Geometry: final body of the model. Coordinates: model frame, mm. Face numbers are marked on the shaded views. A direction names the side the tool comes from. Round coordinates to 2 decimals unless told otherwise and drop trailing zeros. Loops run counter-clockwise (first coordinate to the right, second up) from the corner with the lowest first, then second, coordinate; pieces in that order, holes last. Notation, with made-up numbers: M 82,43 L 119,43 A17 cw 119,59 Z; hole C 44,37 d5. An arc over 180 degrees is marked long. Write each question's results on one line, items separated by ' | '.
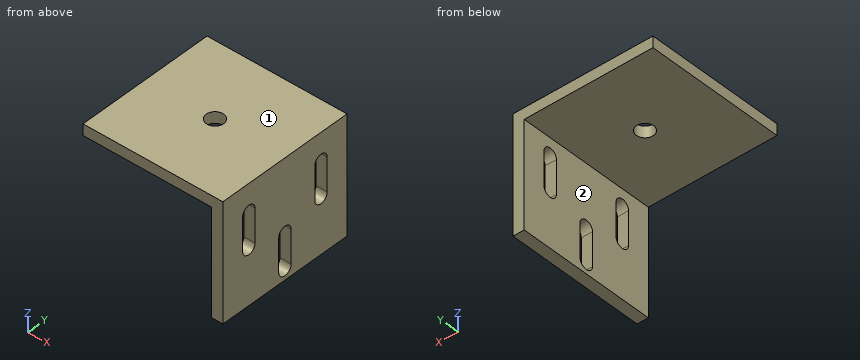
```python
from build123d import *

# Parameters (mm, degrees)
F1_DEPTH = 25
F3_D     = 6.2
F5_DEPTH = 4.001


with BuildPart() as f1:
    # F0 (on Front) → F1 (new body, symmetric)
    with BuildSketch(Plane.XZ):
        Polygon((0, -42), (0, 0), (-50, 0), (-50, -4), (-4, -4), (-4, -42), align=None)
    extrude(amount=F1_DEPTH, both=True)

    # F3 (through all)
    with Locations(Plane.XY):
        with Locations((-25, 0)):
            Hole(F3_D / 2)

    # F4 (on face) → F5 (cut, through all)
    with BuildSketch(Plane(origin=(-4, 0, 0), x_dir=(0, -1, 0), z_dir=(-1, 0, 0))):
        with BuildLine():
            ThreePointArc((-17.034974, -22), (-14.534974, -24.5), (-12.034974, -22))
            Line((-12.034974, -22), (-12.034974, -10))
            ThreePointArc((-12.034974, -10), (-14.534974, -7.5), (-17.034974, -10))
            Line((-17.034974, -10), (-17.034974, -22))
        make_face()
        with BuildLine():
            ThreePointArc((-2.5, -38), (0, -40.5), (2.5, -38))
            Line((2.5, -38), (2.5, -26))
            ThreePointArc((2.5, -26), (0, -23.5), (-2.5, -26))
            Line((-2.5, -26), (-2.5, -38))
        make_face()
        with BuildLine():
            ThreePointArc((12.034974, -22), (14.534974, -24.5), (17.034974, -22))
            Line((17.034974, -22), (17.034974, -10))
            ThreePointArc((17.034974, -10), (14.534974, -7.5), (12.034974, -10))
            Line((12.034974, -10), (12.034974, -22))
        make_face()
    extrude(amount=-F5_DEPTH, mode=Mode.SUBTRACT)


solid = f1.part
```
1. Section A-A (z = -31). Output: boundary loops of the cut face in (x, y).
Answer key:
outline: M -4,-25 L 0,-25 L 0,-2.5 L -4,-2.5 Z; M -4,2.5 L 0,2.5 L 0,25 L -4,25 Z
2. Ray query, probe 1 along Y at (x, z) = (-25, -1.5); probe 2 along Z at (x, y) = (-6.5, 1.5). Return the intervals inside material, ascending.
Answer key:
probe 1: y = -25 to -3.1, 3.1 to 25 | probe 2: z = -4 to 0
3. Section B-B (x = -25). Output: boundary loops of the cut face in (y, z), then the cut area to 3 significant figures.
Answer key:
outline: M -25,-4 L -3.1,-4 L -3.1,0 L -25,0 Z; M 3.1,-4 L 25,-4 L 25,0 L 3.1,0 Z | area: 175 mm²
4. Section D-D (y = 18.5). Output: boundary loops of the cut face in (x, z), then the cut area to 3 significant figures.
Answer key:
outline: M -50,-4 L -4,-4 L -4,-42 L 0,-42 L 0,0 L -50,0 Z | area: 352 mm²
5. Pin query (flat end, axial travel): P1, Ø5, axis at y = -18, z = -12, coming from the -X side; P2, Ø5, axis at x = -25, y = 0, coming from the -Z side; P3, Ø3, axis at x = -6.5, y = -10.5, coming from the -Z side. Return the tip coordinate at first contact, or that it passes through.
Answer key:
P1: stops at x = -4 | P2: passes through | P3: stops at z = -4
6. Access query for the marked faces 1 and 2. Directions: +Z, -Z, +X, -X, +Y, -Y. A direction counts if a zero-diameter tool reaches every point of the face in a straight line with its end or side. Return the directions, or none.
Answer key:
face 1: +Z, +X, -X, +Y, -Y | face 2: -Z, -X, +Y, -Y
7. Section C-C (z = -14). Output: boundary loops of the cut face in (x, y).
Answer key:
outline: M -4,-25 L 0,-25 L 0,-17.03 L -4,-17.03 Z; M -4,-12.03 L 0,-12.03 L 0,12.03 L -4,12.03 Z; M -4,17.03 L 0,17.03 L 0,25 L -4,25 Z
